Here's how the part is built. I have some questions about the finished solid (model axes, mm). A direction names the side the tool comes from. Coordinates: 2 decimals unless noted, no trailing zeros. Loops run counter-clockwise (first coordinate to the right, second up) from the corner with the lowest first, then second, coordinate; pieces in that order, holes last. Notation, with made-up numbers: (85.5, 3) -> (127.5, 3) arc R13 cw to (127.5, 19) -> close; hole circle Ø11 at (-2.5, 16.25). An arc over 180 degrees is marked (long way). Answer as a JSON object with one key per item and string values. Group by question number.
1) I'm going to push flat-ended pins straight in: pin 1 (2 mm diameter, centred on x = -3.5, z = -20.5, fed in from +Y); pin 2 (7 mm diameter, centred on x = -38, z = 20, fed in from +Y); pin 3 (0.6 mm diameter, centred on y = 3.5, z = -2.5, fed in from -X). Where does each tip first touch, or does it pass through?
2) Which directions (+Z, -Z, +X, -X, +Y, -Y) give clear straight access to the entire face, cutting with the end or side of a thin tool? Please do faces 1 (the cylindrical face through (-3.812, -1.213, 0.378)), 2 (the flat face through (9, 45, 0)), 3 (the flat face through (7, 26, 0)).
3) If we mould it in two halves opening along X, with no side actions, what happens to faces 4 (the flat face through (0, 3, 0)), 5 (the cylindrical face through (-20.747, -9.535, 0.121)), 6 (the flat face through (12, 17, -6)), 7 (the cylindrical face through (9.535, 40.727, 0.358))? For each: +X half, -X half, draft (parallel to the pull), parting line (faces both ways), or undercut.
4) I want a section at B-B (z = 20). Count the separate pieces of the cut face and the enclosed holes in it, then the cut area to 3 significant figures.
5) I want a section at A-A (x = -38). Write out the boundary of the cut face in (y, z), then the cut area to 4 significant figures.
6) I want a section at D-D (z = 11). Write out the boundary of the cut face in (x, y).
7) I need wall thicknesses on probe 1 along Y at (x, z) = (9.75, 0); probe 2 along Z at (x, y) = (-38, -9.25); probe 3 along X at (y, z) = (2.5, 4.5). Which ranges of each line are inside material? Lowest first, please. Write a range as [from, to].
8) I want a section at C-C (y = 18). Write out the boundary of the cut face in (x, z), then the cut area to 4 significant figures.
```python
from build123d import *

# Parameters (mm, degrees)
BOSS_EXTRUDE1_DEPTH      = 27
BOSS_EXTRUDE1_DEPTH_BACK = 27
CUT_EXTRUDE1_REACH       = 59
SKETCH2_R                = 2.75
CUT_EXTRUDE2_REACH       = 59
SKETCH3_R                = 2.75


with BuildPart() as part:
    # Sketch1 → Boss-Extrude1 (new body, two sides)
    with BuildSketch(Plane.XY) as boss_extrude1_sk:
        with BuildLine():
            Line((-8, -7), (-3.283882181, -2.283882181))
            ThreePointArc((-3.283882181, -2.283882181), (-3.816774078, -1.196760476), (-4, 0))
            Line((-4, 0), (-2.1, 0))
            ThreePointArc((-2.1, 0), (1.48492424, -1.48492424), (0, 2.1))
            Line((0, 2.1), (0, 4))
            ThreePointArc((0, 4), (1.196760476, 3.816774078), (2.283882181, 3.283882181))
            Line((2.283882181, 3.283882181), (7, 8))
            Line((7, 8), (7, 45))
            Line((7, 45), (12, 45))
            Line((12, 45), (12, -12))
            Line((12, -12), (-45, -12))
            Line((-45, -12), (-45, -7))
            Line((-45, -7), (-8, -7))
        make_face()
    extrude(amount=BOSS_EXTRUDE1_DEPTH)
    extrude(boss_extrude1_sk.sketch, amount=-BOSS_EXTRUDE1_DEPTH_BACK)

    # Sketch2 → Cut-Extrude1 (cut, up to next)
    with BuildSketch(Plane(origin=(12, 0, 0), x_dir=(0, 0, -1), z_dir=(1, 0, 0)), mode=Mode.PRIVATE) as cut_extrude1_sk1:
        with Locations((-20, 38)):
            Circle(SKETCH2_R)
    cut_extrude1_tool1 = extrude(cut_extrude1_sk1.sketch, amount=-CUT_EXTRUDE1_REACH, mode=Mode.PRIVATE) & part.part
    add(cut_extrude1_tool1.solids().sort_by_distance((12, 38, 20))[0], mode=Mode.SUBTRACT)
    # Sketch2 → Cut-Extrude1 (cut, up to next)
    with BuildSketch(Plane(origin=(12, 0, 0), x_dir=(0, 0, -1), z_dir=(1, 0, 0)), mode=Mode.PRIVATE) as cut_extrude1_sk2:
        with Locations((0, 38)):
            Circle(SKETCH2_R)
    cut_extrude1_tool2 = extrude(cut_extrude1_sk2.sketch, amount=-CUT_EXTRUDE1_REACH, mode=Mode.PRIVATE) & part.part
    add(cut_extrude1_tool2.solids().sort_by_distance((12, 38, 0))[0], mode=Mode.SUBTRACT)
    # Sketch2 → Cut-Extrude1 (cut, up to next)
    with BuildSketch(Plane(origin=(12, 0, 0), x_dir=(0, 0, -1), z_dir=(1, 0, 0)), mode=Mode.PRIVATE) as cut_extrude1_sk3:
        with Locations((20, 38)):
            Circle(SKETCH2_R)
    cut_extrude1_tool3 = extrude(cut_extrude1_sk3.sketch, amount=-CUT_EXTRUDE1_REACH, mode=Mode.PRIVATE) & part.part
    add(cut_extrude1_tool3.solids().sort_by_distance((12, 38, -20))[0], mode=Mode.SUBTRACT)
    # Sketch2 → Cut-Extrude1 (cut, up to next)
    with BuildSketch(Plane(origin=(12, 0, 0), x_dir=(0, 0, -1), z_dir=(1, 0, 0)), mode=Mode.PRIVATE) as cut_extrude1_sk4:
        with Locations((-20, 18)):
            Circle(SKETCH2_R)
    cut_extrude1_tool4 = extrude(cut_extrude1_sk4.sketch, amount=-CUT_EXTRUDE1_REACH, mode=Mode.PRIVATE) & part.part
    add(cut_extrude1_tool4.solids().sort_by_distance((12, 18, 20))[0], mode=Mode.SUBTRACT)
    # Sketch2 → Cut-Extrude1 (cut, up to next)
    with BuildSketch(Plane(origin=(12, 0, 0), x_dir=(0, 0, -1), z_dir=(1, 0, 0)), mode=Mode.PRIVATE) as cut_extrude1_sk5:
        with Locations((0, 18)):
            Circle(SKETCH2_R)
    cut_extrude1_tool5 = extrude(cut_extrude1_sk5.sketch, amount=-CUT_EXTRUDE1_REACH, mode=Mode.PRIVATE) & part.part
    add(cut_extrude1_tool5.solids().sort_by_distance((12, 18, 0))[0], mode=Mode.SUBTRACT)
    # Sketch2 → Cut-Extrude1 (cut, up to next)
    with BuildSketch(Plane(origin=(12, 0, 0), x_dir=(0, 0, -1), z_dir=(1, 0, 0)), mode=Mode.PRIVATE) as cut_extrude1_sk6:
        with Locations((20, 18)):
            Circle(SKETCH2_R)
    cut_extrude1_tool6 = extrude(cut_extrude1_sk6.sketch, amount=-CUT_EXTRUDE1_REACH, mode=Mode.PRIVATE) & part.part
    add(cut_extrude1_tool6.solids().sort_by_distance((12, 18, -20))[0], mode=Mode.SUBTRACT)

    # Sketch3 → Cut-Extrude2 (cut, up to next)
    with BuildSketch(Plane.XZ.offset(12), mode=Mode.PRIVATE) as cut_extrude2_sk1:
        with Locations((-38, -20)):
            Circle(SKETCH3_R)
    cut_extrude2_tool1 = extrude(cut_extrude2_sk1.sketch, amount=-CUT_EXTRUDE2_REACH, mode=Mode.PRIVATE) & part.part
    add(cut_extrude2_tool1.solids().sort_by_distance((-38, -12, -20))[0], mode=Mode.SUBTRACT)
    # Sketch3 → Cut-Extrude2 (cut, up to next)
    with BuildSketch(Plane.XZ.offset(12), mode=Mode.PRIVATE) as cut_extrude2_sk2:
        with Locations((-38, 0)):
            Circle(SKETCH3_R)
    cut_extrude2_tool2 = extrude(cut_extrude2_sk2.sketch, amount=-CUT_EXTRUDE2_REACH, mode=Mode.PRIVATE) & part.part
    add(cut_extrude2_tool2.solids().sort_by_distance((-38, -12, 0))[0], mode=Mode.SUBTRACT)
    # Sketch3 → Cut-Extrude2 (cut, up to next)
    with BuildSketch(Plane.XZ.offset(12), mode=Mode.PRIVATE) as cut_extrude2_sk3:
        with Locations((-38, 20)):
            Circle(SKETCH3_R)
    cut_extrude2_tool3 = extrude(cut_extrude2_sk3.sketch, amount=-CUT_EXTRUDE2_REACH, mode=Mode.PRIVATE) & part.part
    add(cut_extrude2_tool3.solids().sort_by_distance((-38, -12, 20))[0], mode=Mode.SUBTRACT)
    # Sketch3 → Cut-Extrude2 (cut, up to next)
    with BuildSketch(Plane.XZ.offset(12), mode=Mode.PRIVATE) as cut_extrude2_sk4:
        with Locations((-18, -20)):
            Circle(SKETCH3_R)
    cut_extrude2_tool4 = extrude(cut_extrude2_sk4.sketch, amount=-CUT_EXTRUDE2_REACH, mode=Mode.PRIVATE) & part.part
    add(cut_extrude2_tool4.solids().sort_by_distance((-18, -12, -20))[0], mode=Mode.SUBTRACT)
    # Sketch3 → Cut-Extrude2 (cut, up to next)
    with BuildSketch(Plane.XZ.offset(12), mode=Mode.PRIVATE) as cut_extrude2_sk5:
        with Locations((-18, 0)):
            Circle(SKETCH3_R)
    cut_extrude2_tool5 = extrude(cut_extrude2_sk5.sketch, amount=-CUT_EXTRUDE2_REACH, mode=Mode.PRIVATE) & part.part
    add(cut_extrude2_tool5.solids().sort_by_distance((-18, -12, 0))[0], mode=Mode.SUBTRACT)
    # Sketch3 → Cut-Extrude2 (cut, up to next)
    with BuildSketch(Plane.XZ.offset(12), mode=Mode.PRIVATE) as cut_extrude2_sk6:
        with Locations((-18, 20)):
            Circle(SKETCH3_R)
    cut_extrude2_tool6 = extrude(cut_extrude2_sk6.sketch, amount=-CUT_EXTRUDE2_REACH, mode=Mode.PRIVATE) & part.part
    add(cut_extrude2_tool6.solids().sort_by_distance((-18, -12, 20))[0], mode=Mode.SUBTRACT)


solid = part.part
```
Determined:
{
 "1": {"pin 1": "y = 0", "pin 2": "y = -7", "pin 3": "x = 0"},
 "2": {"face 1": "+Z, -Z, -X", "face 2": "+Z, -Z, +X, -X, +Y", "face 3": "+Z, -Z, -X, +Y"},
 "3": {"face 4": "-X half", "face 5": "undercut", "face 6": "+X half", "face 7": "draft"},
 "4": {"separate pieces": "5", "enclosed holes": "0", "area": "544 mm^2"},
 "5": {"outline": "(-12, -27) -> (-7, -27) -> (-7, -22.75) -> (-12, -22.75) -> close; (-12, -17.25) -> (-7, -17.25) -> (-7, -2.75) -> (-12, -2.75) -> close; (-12, 2.75) -> (-7, 2.75) -> (-7, 17.25) -> (-12, 17.25) -> close; (-12, 22.75) -> (-7, 22.75) -> (-7, 27) -> (-12, 27) -> close", "area": "187.5 mm^2"},
 "6": {"outline": "(-45, -12) -> (12, -12) -> (12, 45) -> (7, 45) -> (7, 8) -> (2.28, 3.28) arc R4 ccw to (0, 4) -> (0, 2.1) arc R2.1 cw (long way) to (-2.1, 0) -> (-4, 0) arc R4 ccw to (-3.28, -2.28) -> (-8, -7) -> (-45, -7) -> close"},
 "7": {"probe 1": "[-12, 15.25], [20.75, 35.25], [40.75, 45]", "probe 2": "[-27, -22.75], [-17.25, -2.75], [2.75, 17.25], [22.75, 27]", "probe 3": "[0, 12]"},
 "8": {"outline": "(7, -27) -> (12, -27) -> (12, -22.75) -> (7, -22.75) -> close; (7, -17.25) -> (12, -17.25) -> (12, -2.75) -> (7, -2.75) -> close; (7, 2.75) -> (12, 2.75) -> (12, 17.25) -> (7, 17.25) -> close; (7, 22.75) -> (12, 22.75) -> (12, 27) -> (7, 27) -> close", "area": "187.5 mm^2"}
}
